Verification items for the finished model (mm, model axes). A direction names the side the tool comes from. Round coordinates to 2 decimals unless told otherwise and drop trailing zeros. Order: outer loops, then holes, each group sorted by start corner. A loop starts at its lowest first (then second) coordinate and runs counter-clockwise, first axis right, second up.
```python
from build123d import *

# Parameters (mm, degrees)
SALIENTE_EXTRUIR2_DEPTH    = 15
CORTAR_EXTRUIR2_DEPTH      = 28.730849248
CORTAR_EXTRUIR2_DEPTH_BACK = 28.730849248
CROQUIS3_R                 = 1.6
CROQUIS4_W                 = 20
CROQUIS4_H                 = 6.5
CORTAR_EXTRUIR3_DEPTH      = 28.730849248
CORTAR_EXTRUIR4_REACH      = 46.373
CROQUIS5_R                 = 1.6
CORTAR_EXTRUIR5_DEPTH      = 3
CORTAR_EXTRUIR6_DEPTH      = 3
REDONDEO1_R                = 1


with BuildPart() as part:
    # Croquis1 → Saliente-Extruir2 (new body)
    with BuildSketch(Plane(origin=(0, 0, 0), x_dir=(1, 0, 0), z_dir=(0, 1, 0))):
        with BuildLine():
            Line((-12, -20), (12, -20))
            Line((12, -20), (12, 20))
            Line((12, 20), (3.5, 20))
            Line((3.5, 20), (3.5, 8.5))
            ThreePointArc((3.5, 8.5), (0, 5), (-3.5, 8.5))
            Line((-3.5, 8.5), (-3.5, 20))
            Line((-3.5, 20), (-12, 20))
            Line((-12, 20), (-12, -20))
        make_face()
    extrude(amount=SALIENTE_EXTRUIR2_DEPTH)

    # Croquis3 → Cortar-Extruir2 (cut, two sides: drawn at the far end of the back side and taken through both)
    with BuildSketch(Plane(origin=(0, 0, 0), x_dir=(0, 0, -1), z_dir=(1, 0, 0)).offset(-CORTAR_EXTRUIR2_DEPTH_BACK)):
        with Locations((16, 7.5)):
            Circle(CROQUIS3_R)
    extrude(amount=CORTAR_EXTRUIR2_DEPTH + CORTAR_EXTRUIR2_DEPTH_BACK, mode=Mode.SUBTRACT)

    # Croquis4 → Cortar-Extruir3 (cut, through all)
    with BuildSketch(Plane(origin=(0, 15, 0), x_dir=(1, 0, 0), z_dir=(0, 1, 0))):
        with Locations((0, -9.75)):
            Rectangle(CROQUIS4_W, CROQUIS4_H)
    extrude(amount=-CORTAR_EXTRUIR3_DEPTH, mode=Mode.SUBTRACT)

    # Croquis5 → Cortar-Extruir4 (cut, up to next)
    with BuildSketch(Plane.XY.offset(20), mode=Mode.PRIVATE) as cortar_extruir4_sk1:
        with Locations((-5, 10)):
            Circle(CROQUIS5_R)
    cortar_extruir4_tool1 = extrude(cortar_extruir4_sk1.sketch, amount=-CORTAR_EXTRUIR4_REACH, mode=Mode.PRIVATE) & part.part
    # Croquis5 → Cortar-Extruir4 (cut, up to next)
    with BuildSketch(Plane.XY.offset(20), mode=Mode.PRIVATE) as cortar_extruir4_sk2:
        with Locations((5, 10)):
            Circle(CROQUIS5_R)
    cortar_extruir4_tool2 = extrude(cortar_extruir4_sk2.sketch, amount=-CORTAR_EXTRUIR4_REACH, mode=Mode.PRIVATE) & part.part
    add(cortar_extruir4_tool1.solids().sort_by_distance((-5, 10, 20))[0], mode=Mode.SUBTRACT)
    add(cortar_extruir4_tool2.solids().sort_by_distance((5, 10, 20))[0], mode=Mode.SUBTRACT)

    # Croquis6 → Cortar-Extruir5 (cut)
    with BuildSketch(Plane(origin=(0, 0, 13), x_dir=(-1, 0, 0), z_dir=(0, 0, -1))):
        Polygon((-3.383419246, 12.8), (-6.616580754, 12.8), (-8.233161507, 10), (-6.616580754, 7.2), (-3.383419246, 7.2), (-1.766838493, 10), align=None)
        Polygon((6.616580754, 12.8), (3.383419246, 12.8), (1.766838493, 10), (3.383419246, 7.2), (6.616580754, 7.2), (8.233161507, 10), align=None)
    extrude(amount=-CORTAR_EXTRUIR5_DEPTH, mode=Mode.SUBTRACT)

    # Croquis7 → Cortar-Extruir6 (cut)
    with BuildSketch(Plane(origin=(12, 0, 0), x_dir=(0, 0, -1), z_dir=(1, 0, 0))):
        Polygon((17.616580754, 4.7), (19.233161507, 7.5), (17.616580754, 10.3), (14.383419246, 10.3), (12.766838493, 7.5), (14.383419246, 4.7), align=None)
    extrude(amount=-CORTAR_EXTRUIR6_DEPTH, mode=Mode.SUBTRACT)

    # Redondeo1
    # the kernel refuses this fillet: 1 mm, written as the material it takes off along each edge
    with BuildSketch(Plane(origin=(14.5, 0, -20), x_dir=(0, 0, 1), z_dir=(-1, 0, 0)), Plane(origin=(-1, 0, -20), x_dir=(0, 0, 1), z_dir=(-1, 0, 0))) as redondeo1_piece_1:
        with BuildLine():
            CenterArc((REDONDEO1_R, REDONDEO1_R), REDONDEO1_R, 180, 90)
            Line((0, REDONDEO1_R), (0, 0))
            Line((0, 0), (REDONDEO1_R, 0))
        make_face()
    extrude(amount=13.5, mode=Mode.SUBTRACT)
    with BuildSketch(Plane(origin=(12, -2.5, -20), x_dir=(0, 0, 1), z_dir=(0, 1, 0)), Plane(origin=(12, -2.5, 20), x_dir=(-1, 0, 0), z_dir=(0, 1, 0))) as redondeo1_piece_2:
        with BuildLine():
            CenterArc((REDONDEO1_R, -REDONDEO1_R), REDONDEO1_R, 90, 90)
            Line((0, -REDONDEO1_R), (0, 0))
            Line((0, 0), (REDONDEO1_R, 0))
        make_face()
    extrude(amount=20, mode=Mode.SUBTRACT)
    with BuildSketch(Plane(origin=(-12, -2.5, 20), x_dir=(1, 0, 0), z_dir=(0, 1, 0)), Plane(origin=(-12, -2.5, -20), x_dir=(0, 0, 1), z_dir=(0, 1, 0))) as redondeo1_piece_3:
        with BuildLine():
            CenterArc((REDONDEO1_R, REDONDEO1_R), REDONDEO1_R, 180, 90)
            Line((0, REDONDEO1_R), (0, 0))
            Line((0, 0), (REDONDEO1_R, 0))
        make_face()
    extrude(amount=20, mode=Mode.SUBTRACT)
    with BuildSketch(Plane(origin=(-1, 15, -20), x_dir=(0, 0, 1), z_dir=(-1, 0, 0)), Plane(origin=(14.5, 15, -20), x_dir=(0, 0, 1), z_dir=(-1, 0, 0))) as redondeo1_piece_4:
        with BuildLine():
            CenterArc((REDONDEO1_R, -REDONDEO1_R), REDONDEO1_R, 90, 90)
            Line((0, -REDONDEO1_R), (0, 0))
            Line((0, 0), (REDONDEO1_R, 0))
        make_face()
    extrude(amount=13.5, mode=Mode.SUBTRACT)


solid = part.part
```
1) Sectioned sample at B-B on x = 0. Record the cut outline in (y, z).
2) Tool access check on faces 1 (the flat face through (5, 12.8, 14)), 2 (the flat face through (0, 15, 0)), 3 (the flat face through (10.521, 8.92, -13.586)), 4 (the flat face through (-7, 7, -20)), 5 (the flat face through (-10, 8, 10)). Record the directions out of +Z, -Z, +X, -X, +Y, -Y that give a thin tool (end or side, any length) a straight path to the whole face; none if there is none.
3) Go/stop test with a flat-tipped pin: pin 1 Ø4 at (x, y) = (-5, 10) entering from +Z. Record where the tip stops, or that it passes through.
4) Scan lines: probe 1 along Z at (x, y) = (7.1, 7.5); probe 2 along Y at (x, z) = (-10, -16); probe 3 along Y at (x, z) = (-5, 17.4). Record each from-to range of solid material in increasing order.
5) Sectioned sample at C-C on z = -9. Record the cut outline in (x, y).
6) Sectioned sample at A-A on x = -9.25. Record the cut outline in (y, z).
7) Draft check along Z on faces 6 (the flat face through (2.564, 11.38, 14.479)), 7 (the cylindrical face through (0, 7, -5)), 8 (the flat face through (11, 10.3, -16)), 9 (the flat face through (-3.5, 7, -14)). Enter one of: released by +Z, released by -Z, zero draft, split by the parting line, or undercut.
Returned:
1. outline: (0, -5) - (15, -5) - (15, 6.5) - (0, 6.5) - close; (0, 13) - (15, 13) - (15, 20) - (0, 20) - close
2. face 1: none
2. face 2: +Z, -Z, +X, -X, +Y
2. face 3: +X
2. face 4: -Z, +X, -X, +Y, -Y
2. face 5: +Y, -Y
3. pin 1: stops at z = 20
4. probe 1: z = -20 to -17.6, -14.4 to 6.5, 13 to 20
4. probe 2: y = 0 to 5.9, 9.1 to 15
4. probe 3: y = 0 to 8.4, 11.6 to 15
5. outline: (-12, 0) - (-3.5, 0) - (-3.5, 15) - (-12, 15) - close; (3.5, 0) - (12, 0) - (12, 15) - (3.5, 15) - close
6. outline: (0, -19) arc R1 ccw to (1, -20) - (14, -20) arc R1 ccw to (15, -19) - (15, 6.5) - (0, 6.5) - close; (0, 13) - (15, 13) - (15, 20) - (0, 20) - close; hole circle Ø3.2 at (7.5, -16)
7. face 6: undercut
7. face 7: released by -Z
7. face 8: undercut
7. face 9: zero draft
